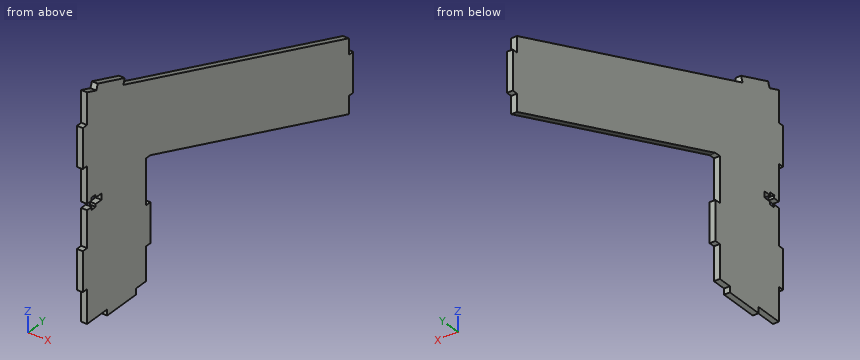
```python
from build123d import *

# Parameters (mm, degrees)
BOSS_EXTRUDE1_DEPTH = 3
CUT_EXTRUDE1_DEPTH  = 267.131484195
SKETCH3_W           = 29.976768642
SKETCH3_H           = 52.268511193
CUT_EXTRUDE2_DEPTH  = 233.651187464
SKETCH5_W           = 11.091910703
SKETCH5_H           = 3
SKETCH5_W_2         = 10
CUT_EXTRUDE4_DEPTH  = 224.001992956
SKETCH6_W           = 20
SKETCH6_H           = 3
CUT_EXTRUDE5_DEPTH  = 224.001992956
SKETCH7_W           = 40
SKETCH7_H           = 3
CUT_EXTRUDE6_DEPTH  = 224.001992956
CUT_EXTRUDE7_REACH  = 225.002
SKETCH8_W           = 20
SKETCH8_H           = 3
CUT_EXTRUDE8_REACH  = 225.002
SKETCH9_W           = 22.898992834
SKETCH9_H           = 3
SKETCH10_W          = 3
SKETCH10_H          = 7
SKETCH10_H_2        = 13.984631039
CUT_EXTRUDE9_DEPTH  = 224.001992956
CUT_EXTRUDE10_DEPTH = 10
SKETCH13_W          = 3
SKETCH13_H          = 20
BOSS_EXTRUDE2_DEPTH = 3
CUT_EXTRUDE11_REACH = 225.002
SKETCH14_W          = 3.1
SKETCH14_H          = 10
SKETCH15_W          = 6
SKETCH15_H          = 2.8
CUT_EXTRUDE12_DEPTH = 224.001992956
SKETCH16_R          = 0.05
CUT_EXTRUDE13_DEPTH = 224.001992956
SKETCH17_R          = 0.05
CUT_EXTRUDE14_DEPTH = 10


with BuildPart() as part:
    # Sketch1 → Boss-Extrude1 (new body)
    with BuildSketch(Plane(origin=(0, 0, 0), x_dir=(0, 0, -1), z_dir=(1, 0, 0))):
        Polygon((0, 0), (120, 0), (188.404028665, 187.938524157), (68.404028665, 187.938524157), align=None)
    extrude(amount=BOSS_EXTRUDE1_DEPTH)

    # Sketch2 → Cut-Extrude1 (cut, through all)
    with BuildSketch(Plane(origin=(3, 0, 0), x_dir=(0, 0, -1), z_dir=(1, 0, 0))):
        Polygon((188.404028665, 187.938524157), (137.101007166, 46.984631039), (57.101007166, 46.984631039), (108.404028665, 187.938524157), align=None)
    extrude(amount=-CUT_EXTRUDE1_DEPTH, mode=Mode.SUBTRACT)

    # Sketch3 → Cut-Extrude2 (cut, through all)
    with BuildSketch(Plane(origin=(3, 0, 0), x_dir=(0, 0, -1), z_dir=(1, 0, 0))):
        with Locations((134.988384321, 26.134255597)):
            Rectangle(SKETCH3_W, SKETCH3_H)
    extrude(amount=-CUT_EXTRUDE2_DEPTH, mode=Mode.SUBTRACT)

    # Sketch5 → Cut-Extrude4 (cut, through all)
    with BuildSketch(Plane(origin=(3, 0, 0), x_dir=(0, 0, -1), z_dir=(1, 0, 0))):
        with Locations((72.858073314, 186.438524157)):
            Rectangle(SKETCH5_W, SKETCH5_H)
        with Locations((103.404028665, 186.438524157)):
            Rectangle(SKETCH5_W_2, SKETCH5_H)
    extrude(amount=-CUT_EXTRUDE4_DEPTH, mode=Mode.SUBTRACT)

    # Sketch6 → Cut-Extrude5 (cut, through all)
    with BuildSketch(Plane(origin=(3, 0, 0), x_dir=(0, 0, -1), z_dir=(1, 0, 0))):
        with Locations((110, 1.5)):
            Rectangle(SKETCH6_W, SKETCH6_H)
        with Locations((10, 1.5)):
            Rectangle(SKETCH6_W, SKETCH6_H)
    extrude(amount=-CUT_EXTRUDE5_DEPTH, mode=Mode.SUBTRACT)

    # Sketch7 → Cut-Extrude6 (cut, through all)
    with BuildSketch(Plane(origin=(3, 0, 0), x_dir=(0, 0, -1), z_dir=(1, 0, 0))):
        with Locations((60, 1.5)):
            Rectangle(SKETCH7_W, SKETCH7_H)
    extrude(amount=-CUT_EXTRUDE6_DEPTH, mode=Mode.SUBTRACT)

    # Sketch8 → Cut-Extrude7 (cut, up to next)
    with BuildSketch(Plane(origin=(3, 0, 0), x_dir=(0, 0, -1), z_dir=(1, 0, 0)), mode=Mode.PRIVATE) as cut_extrude7_sk1:
        with Locations((110, 45.484631039)):
            Rectangle(SKETCH8_W, SKETCH8_H)
    cut_extrude7_tool1 = extrude(cut_extrude7_sk1.sketch, amount=-CUT_EXTRUDE7_REACH, mode=Mode.PRIVATE) & part.part
    add(cut_extrude7_tool1.solids().sort_by_distance((3, 45.484631, -110))[0], mode=Mode.SUBTRACT)

    # Sketch9 → Cut-Extrude8 (cut, up to next)
    with BuildSketch(Plane(origin=(3, 0, 0), x_dir=(0, 0, -1), z_dir=(1, 0, 0)), mode=Mode.PRIVATE) as cut_extrude8_sk1:
        with Locations((68.550503583, 45.484631039)):
            Rectangle(SKETCH9_W, SKETCH9_H)
    cut_extrude8_tool1 = extrude(cut_extrude8_sk1.sketch, amount=-CUT_EXTRUDE8_REACH, mode=Mode.PRIVATE) & part.part
    add(cut_extrude8_tool1.solids().sort_by_distance((3, 45.484631, -68.550504))[0], mode=Mode.SUBTRACT)

    # Sketch10 → Cut-Extrude9 (cut, through all)
    with BuildSketch(Plane(origin=(3, 0, 0), x_dir=(0, 0, -1), z_dir=(1, 0, 0))):
        with Locations((118.5, 40.484631039)):
            Rectangle(SKETCH10_W, SKETCH10_H)
        with Locations((118.5, 9.992315519)):
            Rectangle(SKETCH10_W, SKETCH10_H_2)
    extrude(amount=-CUT_EXTRUDE9_DEPTH, mode=Mode.SUBTRACT)

    # Sketch11 → Cut-Extrude10 (cut)
    with BuildSketch(Plane(origin=(3, 0, 0), x_dir=(0, 0, -1), z_dir=(1, 0, 0))):
        Polygon((67.312117962, 184.938524157), (1.091910703, 3), (4.091910703, 3), (70.312117962, 184.938524157), align=None)
    extrude(amount=-CUT_EXTRUDE10_DEPTH, mode=Mode.SUBTRACT)

    # Sketch13 → Boss-Extrude2 (add)
    with BuildSketch(Plane(origin=(0, -0.964181415, -2.649066665), x_dir=(1, 0, 0), z_dir=(0, 0.3420201433256657, 0.9396926207859095))):
        with Locations((1.5, 21.02606043)):
            Rectangle(SKETCH13_W, SKETCH13_H)
    extrude(amount=BOSS_EXTRUDE2_DEPTH)

    # Sketch14 → Cut-Extrude11 (cut, up to next)
    with BuildSketch(Plane(origin=(3, 0, 0), x_dir=(0, 0, -1), z_dir=(1, 0, 0)), mode=Mode.PRIVATE) as cut_extrude11_sk1:
        with Locations((60, 8)):
            Rectangle(SKETCH14_W, SKETCH14_H)
    cut_extrude11_tool1 = extrude(cut_extrude11_sk1.sketch, amount=-CUT_EXTRUDE11_REACH, mode=Mode.PRIVATE) & part.part
    add(cut_extrude11_tool1.solids().sort_by_distance((3, 8, -60))[0], mode=Mode.SUBTRACT)

    # Sketch15 → Cut-Extrude12 (cut, through all)
    with BuildSketch(Plane(origin=(3, 0, 0), x_dir=(0, 0, -1), z_dir=(1, 0, 0))):
        with Locations((59.96, 7.6)):
            Rectangle(SKETCH15_W, SKETCH15_H)
    extrude(amount=-CUT_EXTRUDE12_DEPTH, mode=Mode.SUBTRACT)

    # Sketch16 → Cut-Extrude13 (cut, through all)
    with BuildSketch(Plane(origin=(3, 0, 0), x_dir=(0, 0, -1), z_dir=(1, 0, 0))):
        with Locations((56.96, 6.2)):
            Circle(SKETCH16_R)
    extrude(amount=-CUT_EXTRUDE13_DEPTH, mode=Mode.SUBTRACT)

    # Sketch17 → Cut-Extrude14 (cut)
    with BuildSketch(Plane(origin=(3, 0, 0), x_dir=(0, 0, -1), z_dir=(1, 0, 0))):
        with Locations((62.96, 6.2)):
            Circle(SKETCH17_R)
    extrude(amount=-CUT_EXTRUDE14_DEPTH, mode=Mode.SUBTRACT)


solid = part.part
```
CAD build for the part. Positions are in the model's coordinates, mm. Give positions to 0.01 mm unless a question says otherwise; leave off trailing zeros. Order: outer loops, then holes, each group sorted by start corner. A loop starts at its lowest first (then second) coordinate and runs counter-clockwise, first axis right, second up.
(1) Flat gauge pins, fed straight in: pin 1 (0.9 mm diameter, centred on x = 1.5, y = 1.5, fed in from -Z); pin 2 (1.5 mm diameter, centred on x = 1.5, y = 59, fed in from +Z); pin 3 (1.5 mm diameter, centred on x = 2, z = -100.5, fed in from +Y). Where does each tip first touch, or does it go through?
(2) Drill centre lines: L1, parallel to Z at x = 1.2, y = 66; L2, parallel to Z at x = 0.3, y = 140; L3, parallel to Y at x = 2.1, z = -12.5. Where is each one in solid material? Low to high.
(3) Saw through at B-B, the plane y = 168.5. Give the cut face in (x, z).
(4) Saw through at A-A, the plane z = -68.5. Give the cut face in (x, y).
(5) Saw through at C-C, the plane z = -17.5. Give the cut face in (x, y).
Results found:
1. pin 1: stops at z = -100
1. pin 2: stops at z = -24.2
1. pin 3: stops at y = 184.94
2. L1: z = -64.02 to -27.02
2. L2: z = -90.96 to -53.96
2. L3: y = 3 to 28.47
3. outline: (0, -101.33) - (3, -101.33) - (3, -64.33) - (0, -64.33) - close
4. outline: (0, 3) - (3, 3) - (3, 43.98) - (0, 43.98) - close; (0, 78.3) - (3, 78.3) - (3, 179.96) - (0, 179.96) - close
5. outline: (0, 3) - (3, 3) - (3, 39.84) - (0, 39.84) - close
